Source: CAD feature listing. Evaluate the final solid. Frame: model axes, mm. A direction names the side the tool comes from. Coordinates: 2 decimals unless noted, no trailing zeros. Write each loop counter-clockwise with the first axis right and the second up, starting at its lowest first coordinate (ties: lowest second). Pieces come first, ordered by that corner, then holes. Notation, with made-up numbers: (64.25, 29.25) - (74.25, 29.25) arc R22 ccw to (74.25, 48.25) - close; hole circle Ø9 at (54.25, -29.75). An arc over 180 degrees is marked (long way). One line per item, written item: value.
from build123d import *

# Parameters (mm, degrees)
SKETCH1_R           = 2.54
BOSS_EXTRUDE1_DEPTH = 0.635
SKETCH2_R           = 3.81
SKETCH2_R_2         = 2.54
BOSS_EXTRUDE2_DEPTH = 4.7752


with BuildPart() as part:
    # Sketch1 → Boss-Extrude1 (new body)
    with BuildSketch(Plane.XY):
        with BuildLine():
            ThreePointArc((-1.7859375, 4.116609732), (-9.8425, 0), (-1.7859375, -4.116609732))
            ThreePointArc((-1.7859375, -4.116609732), (0, -3.538575571), (1.7859375, -4.116609732))
            ThreePointArc((1.7859375, -4.116609732), (9.8425, 0), (1.7859375, 4.116609732))
            ThreePointArc((1.7859375, 4.116609732), (0, 3.538575571), (-1.7859375, 4.116609732))
        make_face()
        with Locations((-4.7625, 0)):
            Circle(SKETCH1_R, mode=Mode.SUBTRACT)
        with Locations((4.7625, 0)):
            Circle(SKETCH1_R, mode=Mode.SUBTRACT)
    boss_extrude1 = extrude(amount=BOSS_EXTRUDE1_DEPTH)

    # Sketch2 → Boss-Extrude2 (add)
    with BuildSketch(Plane.XY.offset(0.635)):
        with Locations((-4.7625, 0)):
            Circle(SKETCH2_R)
        with Locations((-4.7625, 0)):
            Circle(SKETCH2_R_2, mode=Mode.SUBTRACT)
    boss_extrude2 = extrude(amount=BOSS_EXTRUDE2_DEPTH)

    # Mirror1: Boss-Extrude2 across plane
    add(boss_extrude2.mirror(Plane(origin=(0, 0, 0), x_dir=(0, 0, 1), z_dir=(1, 0, 0))))

    # Mirror2: Boss-Extrude1 across plane
    add(boss_extrude1.mirror(Plane.XY.offset(3.0226)))


solid = part.part
1) Section query B-B on x = -5.75. Output: boundary loops of the cut face in (y, z) (3 decimals).
Values found:
outline: (-4.983, 0) - (-2.34, 0) - (-2.34, 6.045) - (-4.983, 6.045) - (-4.983, 5.41) - (-3.68, 5.41) - (-3.68, 0.635) - (-4.983, 0.635) - close; (2.34, 0) - (4.983, 0) - (4.983, 0.635) - (3.68, 0.635) - (3.68, 5.41) - (4.983, 5.41) - (4.983, 6.045) - (2.34, 6.045) - close
2) Material intervals for line 1 (Z direction, x = 8.5, y = 2.5) (3 decimals); line 2 (X direction, y = -1, z = 2.25); line 3 (X direction, y = -1.75, z = 1.5), sorted ascending.
Values found:
line 1: 0 to 0.635, 5.41 to 6.045
line 2: -8.44 to -7.1, -2.43 to -1.09, 1.09 to 2.43, 7.1 to 8.44
line 3: -8.15 to -6.6, -2.92 to -1.38, 1.38 to 2.92, 6.6 to 8.15
3) Reachability of faces 4 (the cylindrical face through (-9.84, 0.16, 0.31)), 5 (the flat face through (0, 0, 5.41)) from +Z, -Z, +X, -X, +Y, -Y: full face, straight path, thin tool, end or side. Return the list, or none.
Values found:
face 4: +Z, -Z
face 5: none
4) Section query D-D on z = 1.25. Output: boundary loops of the cut face in (x, y).
Values found:
outline: circle Ø7.62 at (-4.76, 0); circle Ø7.62 at (4.76, 0); hole circle Ø5.08 at (-4.76, 0); hole circle Ø5.08 at (4.76, 0)
5) Draft query along Z for faces 1 (the flat face through (0, 0, 6.045)), 2 (the cylindrical face through (9.84, -0.16, 5.73)), 3 (the cylindrical face through (8.57, 0.17, 2.99)). Return one class per face: released by +Z, released by -Z, zero draft, split by the parting line, or undercut.
Values found:
face 1: released by +Z
face 2: zero draft
face 3: undercut
6) Section query C-C on z = 5.75. Output: boundary loops of the cut face in (x, y).
Values found:
outline: (-1.79, -4.12) arc R3.05 cw to (1.79, -4.12) arc R5.08 ccw (long way) to (1.79, 4.12) arc R3.05 cw to (-1.79, 4.12) arc R5.08 ccw (long way) to start; hole circle Ø5.08 at (-4.76, 0); hole circle Ø5.08 at (4.76, 0)
7) Contact query for flat-ended pins moving along their axis: P1, Ø4.5, axis at x = 4.76, y = 0, coming from the +Z side; P2, Ø1, axis at x = -5, z = 2.5, coming from the +Y side. Output: stop coordinate, or through.
Values found:
P1: through
P2: y = 3.81
8) Section query A-A on y = 0. Output: boundary loops of the cut face in (x, z) (1 decimal), then the cut area to 3 significant figures.
Values found:
outline: (-9.8, 0) - (-7.3, 0) - (-7.3, 6) - (-9.8, 6) - (-9.8, 5.4) - (-8.6, 5.4) - (-8.6, 0.6) - (-9.8, 0.6) - close; (-2.2, 0) - (2.2, 0) - (2.2, 6) - (-2.2, 6) - close; (7.3, 0) - (9.8, 0) - (9.8, 0.6) - (8.6, 0.6) - (8.6, 5.4) - (9.8, 5.4) - (9.8, 6) - (7.3, 6) - close; hole (-1, 0.6) - (1, 0.6) - (1, 5.4) - (-1, 5.4) - close
area: 36.4 mm2
